from build123d import *

# Parameters (mm, degrees)
BOSS_EXTRUDE1_DEPTH  = 76.2
M4_CLEARANCE_HOLE1_D = 4.3
SKETCH2_R            = 5.5
CUT_EXTRUDE1_DEPTH   = 8.636
SKETCH6_R            = 4.35
CUT_EXTRUDE2_DEPTH   = 13.97
CUT_EXTRUDE3_REACH   = 114.405
SKETCH7_R            = 3.175


with BuildPart() as part:
    # Sketch1 → Boss-Extrude1 (new body)
    with BuildSketch(Plane.XY):
        Polygon((-35.999033751, 18.830418264), (-35.999033751, -25.619581736), (33.850966249, -25.619581736), (33.850966249, -31.969581736), (-42.349033751, -31.969581736), (-42.349033751, 18.830418264), align=None)
    extrude(amount=BOSS_EXTRUDE1_DEPTH)

    # M4 Clearance Hole1 (through all)
    with Locations(Plane(origin=(-35.999033751, 0, 0), x_dir=(0, 0, -1), z_dir=(1, 0, 0))):
        with Locations((-30.154792935, 14.695211199), (-30.154792935, -10.054374671), (-5.405207065, -10.054374671), (-5.405207065, 14.695211199)):
            Hole(M4_CLEARANCE_HOLE1_D / 2)

    # Sketch2 → Cut-Extrude1 (cut)
    with BuildSketch(Plane(origin=(-35.999033751, 0, 0), x_dir=(0, 0, -1), z_dir=(1, 0, 0))):
        with Locations((-17.78, 2.320418264)):
            Circle(SKETCH2_R)
    extrude(amount=-CUT_EXTRUDE1_DEPTH, mode=Mode.SUBTRACT)

    # Sketch6 → Cut-Extrude2 (cut)
    with BuildSketch(Plane.XZ.offset(31.969581736)):
        with Locations(Location((16.591266249, 65, 0), (0, 0, 270))):
            Circle(SKETCH6_R)
        with Locations(Location((16.591266249, 15, 0), (0, 0, 270))):
            Circle(SKETCH6_R)
        with Locations(Location((16.591266249, 40, 0), (0, 0, 270))):
            Circle(SKETCH6_R)
    extrude(amount=-CUT_EXTRUDE2_DEPTH, mode=Mode.SUBTRACT)

    # Sketch7 → Cut-Extrude3 (cut, up to next)
    with BuildSketch(Plane.ZY.offset(42.349033751), mode=Mode.PRIVATE) as cut_extrude3_sk1:
        with Locations(Location((53.975, 6.130418264, 0), (0, 0, 270))):
            Circle(SKETCH7_R)
    cut_extrude3_tool1 = extrude(cut_extrude3_sk1.sketch, amount=-CUT_EXTRUDE3_REACH, mode=Mode.PRIVATE) & part.part
    # Sketch7 → Cut-Extrude3 (cut, up to next)
    with BuildSketch(Plane.ZY.offset(42.349033751), mode=Mode.PRIVATE) as cut_extrude3_sk2:
        with Locations(Location((66.675, 6.130418264, 0), (0, 0, 270))):
            Circle(SKETCH7_R)
    cut_extrude3_tool2 = extrude(cut_extrude3_sk2.sketch, amount=-CUT_EXTRUDE3_REACH, mode=Mode.PRIVATE) & part.part
    add(cut_extrude3_tool1.solids().sort_by_distance((-42.349034, 6.130418, 53.975))[0], mode=Mode.SUBTRACT)
    add(cut_extrude3_tool2.solids().sort_by_distance((-42.349034, 6.130418, 66.675))[0], mode=Mode.SUBTRACT)


solid = part.part
The listing builds one solid part. Answer for the finished solid, in the listing's coordinates (mm). A direction names the side the tool comes from. Round coordinates to 2 decimals unless told otherwise and drop trailing zeros. Order: outer loops, then holes, each group sorted by start corner. A loop starts at its lowest first (then second) coordinate and runs counter-clockwise, first axis right, second up. Notation, with made-up numbers: M 12.5,18.25 L 34.5,18.25 A32 cw 34.5,53.25 Z; hole C 0,23 d1. An arc over 180 degrees is marked long. Answer in a Markdown table with one row per item. Add a question column.
1) Which of the six approach directions +Z, -Z, +X, -X, +Y, -Y give full straight-line access (tool end or side, diameter ignored) to faces 1 (the face through (-35.999, -3, 38)), 2 (the face through (-39.218, 6.819, 50.876))?
2) Consider line 1 along X through (y, z) = (-29, 40); line 2 along Y through (x, z) = (14.5, 19.5); line 3 along X through (y, z) = (-6, 24). Determine where each line is inside the solid, lowest interval first. Write a range as from..to.
3) The part is cut by section A-A on z = 40. Determine the outline of the cut face in (x, y).
4) The part is cut by section D-D on y = -21.5. Determine the outline of the cut face in (x, z), plus the area to 3 significant figures.
5) The part is cut by section B-B on z = 17.78. Determine the outline of the cut face in (x, y), plus the area to 3 significant figures.
6) The part is cut by section C-C on x = -16. Determine the outline of the cut face in (y, z).
7) Determine the mould class of faces 3 (the face through (-39, 18.83, 38)), 4 (the face through (33.851, -29, 38)), 5 (the face through (12.732, -28.839, 12.993)) for opening direction X: pulls with the +X half, pulls with the -X half, needs draft (parallel to the pull), parting line crosses it, or undercut.
8) Flat-ended cylindrical pins translate along their axes: pin 1 Ø1 at (x, z) = (22.5, 50.5) entering from +Y; pin 2 Ø7 at (x, z) = (16.59, 65) entering from -Y; pin 3 Ø7.5 at (y, z) = (6.13, 53.98) entering from +X. Find the tip coordinate at first contact, or state that the pin passes through.
Findings below:
| question | item | result |
|---|---|---|
| 1 | face 1 | +Z, -Z, +X, +Y |
| 1 | face 2 | +X, -X |
| 2 | line 1 | x = -42.35..12.24, 20.94..33.85 |
| 2 | line 2 | y = -31.97..-25.62 |
| 2 | line 3 | x = -42.35..-36 |
| 3 | outline | M -42.35,-31.97 L 12.24,-31.97 L 12.24,-25.62 L -36,-25.62 L -36,18.83 L -42.35,18.83 Z; M 20.94,-31.97 L 33.85,-31.97 L 33.85,-25.62 L 20.94,-25.62 Z |
| 4 | outline | M -42.35,0 L -36,0 L -36,76.2 L -42.35,76.2 Z |
| 4 | area | 484 mm² |
| 5 | outline | M -42.35,-31.97 L 13.25,-31.97 L 13.25,-25.62 L -36,-25.62 L -36,-3.18 L -42.35,-3.18 Z; M -42.35,7.82 L -36,7.82 L -36,18.83 L -42.35,18.83 Z; M 19.94,-31.97 L 33.85,-31.97 L 33.85,-25.62 L 19.94,-25.62 Z |
| 5 | area | 654 mm² |
| 6 | outline | M -31.97,0 L -25.62,0 L -25.62,76.2 L -31.97,76.2 Z |
| 7 | face 3 | needs draft |
| 7 | face 4 | pulls with the +X half |
| 7 | face 5 | undercut |
| 8 | pin 1 | stops at y = -25.62 |
| 8 | pin 2 | passes through |
| 8 | pin 3 | stops at x = -36 |
